from build123d import *

# Parameters (mm, degrees)
SKETCH1_W           = 300
SKETCH1_H           = 250
SKETCH1_R           = 2
BOSS_EXTRUDE1_DEPTH = 5
SKETCH2_W           = 100
SKETCH2_H           = 185
CUT_EXTRUDE1_DEPTH  = 6
FILLET1_R           = 20


with BuildPart() as part:
    # Sketch1 → Boss-Extrude1 (new body)
    with BuildSketch(Plane(origin=(0, 0, 0), x_dir=(1, 0, 0), z_dir=(0, 1, 0))):
        Rectangle(SKETCH1_W, SKETCH1_H)
        with Locations((-140, -115)):
            Circle(SKETCH1_R, mode=Mode.SUBTRACT)
        with Locations((-140, 115)):
            Circle(SKETCH1_R, mode=Mode.SUBTRACT)
        with Locations((140, -115)):
            Circle(SKETCH1_R, mode=Mode.SUBTRACT)
        with Locations((140, 115)):
            Circle(SKETCH1_R, mode=Mode.SUBTRACT)
    extrude(amount=BOSS_EXTRUDE1_DEPTH)

    # Sketch2 → Cut-Extrude1 (cut, through all)
    with BuildSketch(Plane(origin=(0, 5, 0), x_dir=(1, 0, 0), z_dir=(0, 1, 0))):
        with Locations((0, 32.5)):
            Rectangle(SKETCH2_W, SKETCH2_H)
    extrude(amount=-CUT_EXTRUDE1_DEPTH, mode=Mode.SUBTRACT)

    # Fillet1
    fillet1_edges = [part.edges().sort_by_distance(p)[0] for p in [
        (-50, 2.5, 60),
        (50, 2.5, 60),
    ]]
    fillet(fillet1_edges, radius=FILLET1_R)


solid = part.part
The model under review builds one solid part; all positions refer to its coordinate system, in mm. A direction names the side the tool comes from. Round coordinates to 2 decimals unless told otherwise and drop trailing zeros. Order: outer loops, then holes, each group sorted by start corner. A loop starts at its lowest first (then second) coordinate and runs counter-clockwise, first axis right, second up. Notation, with made-up numbers: (-19, 1.25) -> (0, 1.25) arc R21 cw to (0, 34.25) -> close; hole circle Ø5 at (7, 70). An arc over 180 degrees is marked (long way). Write item = value, one per line. Start each with the question number.
Item 1: For line 1 along Z through (x, y) = (-140, 1.55); line 2 along X through (y, z) = (1.4, 115); line 3 along X through (y, z) = (2.1, -115), list the stretches that pass through material, from the lowest coordinate up.
Item 2: Consider section C-C on x = 17. Write out the cut boundary in (y, z), plus the area to 3 significant figures.
Item 3: Consider section D-D on x = -45.5. Write out the cut boundary in (y, z).
Item 4: Clearance check with a flat-ended pin moving along its axis: pin 1 Ø3 at (x, z) = (-140, 115) entering from -Y. State where the tip first meets the part, or that it passes through.
Item 5: Consider section A-A on y = 2.2. Write out the cut boundary in (x, z), plus the area to 3 significant figures.
Item 6: For faces 1 (the face through (-69, 0, -2)), 2 (the face through (-44.297, 2.465, 53.986)), list the 3-axis set-ups (+Z, -Z, +X, -X, +Y, -Y) from which the entire face can be reached by the end or side of a thin tool; tool diameter is ignored.
Item 7: Consider section B-B on z = 31. Write out the cut boundary in (x, y), plus the area to 3 significant figures.
Conclusion:
q1.line_1 = -125 to -117, -113 to 113, 117 to 125
q1.line_2 = -150 to -142, -138 to 138, 142 to 150
q1.line_3 = -150 to -142, -138 to -50, 50 to 138, 142 to 150
q2.outline = (0, 60) -> (5, 60) -> (5, 125) -> (0, 125) -> close
q2.area = 325 mm2
q3.outline = (0, 52.64) -> (5, 52.64) -> (5, 125) -> (0, 125) -> close
q4.pin_1 = through
q5.outline = (-150, -125) -> (-50, -125) -> (-50, 40) arc R20 cw to (-30, 60) -> (30, 60) arc R20 cw to (50, 40) -> (50, -125) -> (150, -125) -> (150, 125) -> (-150, 125) -> close; hole circle Ø4 at (-140, -115); hole circle Ø4 at (-140, 115); hole circle Ø4 at (140, -115); hole circle Ø4 at (140, 115)
q5.area = 56,600 mm2
q6.face_1 = +Z, -Z, +X, -X, -Y
q6.face_2 = -Z, +Y, -Y
q7.outline = (-150, 0) -> (-50, 0) -> (-50, 5) -> (-150, 5) -> close; (50, 0) -> (150, 0) -> (150, 5) -> (50, 5) -> close
q7.area = 1,000 mm2
